Read the model definition and answer for the solid it produces. Units are mm, in the model's axes. Face numbers are marked on the shaded views. A direction names the side the tool comes from. Round coordinates to 2 decimals unless told otherwise and drop trailing zeros. Order: outer loops, then holes, each group sorted by start corner. A loop starts at its lowest first (then second) coordinate and runs counter-clockwise, first axis right, second up. Notation, with made-up numbers: (59, 61.5) -> (93, 61.5) arc R13 ccw to (93, 80.5) -> close; hole circle Ø9 at (74.5, -0.75). An arc over 180 degrees is marked (long way). Use a Markdown table: item, result. Add a question column.
1. For the marked faces 5, 6, 7, 8 and 9, determine the directions among +Z, -Z, +X, -X, +Y, -Y from which every point of the face is accessible in a straight line to the end or side of a thin tool.
2. Given pin 1 (1.2 mm diameter, centred on x = 6, z = 2.5, fed in from +Y); pin 2 (0.9 mm diameter, centred on x = 3.5, z = 3, fed in from +Y); pin 3 (1.2 mm diameter, centred on x = 14, z = 2.5, fed in from +Y), each flat-ended and moving along its own axis, determine where each tip first touches the part or whether it passes through.
3. Section B-B, the plane z = 3 is taken. Give the vertices of the cut face in (x, y).
4. The mould has two halves that part along X. Classify the marked faces 1, 2, 3 and 4: +X half, -X half, draft (parallel to the pull), parting line (faces both ways), or undercut.
5. Section D-D, the plane y = 15.25 is taken. Give the vertices of the cut face in (x, z).
6. Section A-A, the plane y = 10.75 is taken. Give the vertices of the cut face in (x, z).
7. Consider L1, parallel to X at y = 9.25, z = 0.95; L2, parallel to Y at x = 6.25, z = 1.6; L3, parallel to Y at x = 9, z = 3.2. Determine where each line is inside the solid, lowest interval first. Write a range as [from, to].
8. Section C-C, the plane x = 4 is taken. Give the vertices of the cut face in (y, z).
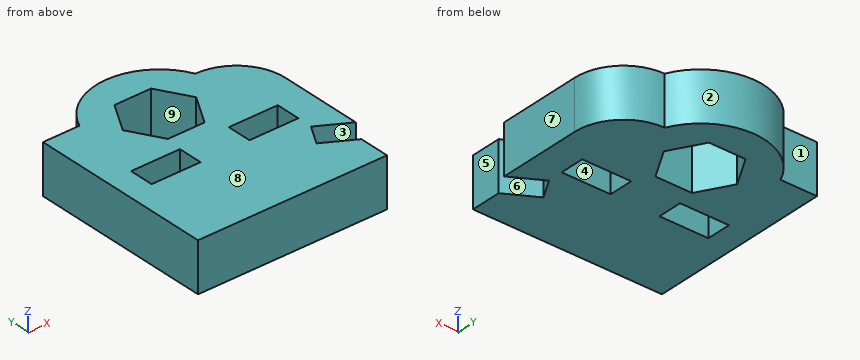
```python
from build123d import *

# Parameters (mm, degrees)
SKETCH1_W           = 4
SKETCH1_H           = 2
BOSS_EXTRUDE1_DEPTH = 4


with BuildPart() as part:
    # Sketch1 → Boss-Extrude1 (new body)
    with BuildSketch(Plane.XY):
        with BuildLine():
            Line((14.475572066, 6), (15.475572066, 7.732050808))
            Line((15.475572066, 7.732050808), (17.939673681, 6.309401077))
            Line((17.939673681, 6.309401077), (17.939673681, 13.142551265))
            ThreePointArc((17.939673681, 13.142551265), (16.768100806, 15.97097839), (13.939673681, 17.142551265))
            ThreePointArc((13.939673681, 17.142551265), (9.2, 20.197069168), (4.460326319, 17.142551265))
            Line((4.460326319, 17.142551265), (1.48, 17.142551265))
            Line((1.48, 17.142551265), (1.48, 2.09107808))
            Line((1.48, 2.09107808), (16.939673681, 2.09107808))
            Line((16.939673681, 2.09107808), (16.939673681, 4.577350269))
            Line((16.939673681, 4.577350269), (14.475572066, 6))
        make_face()
        with Locations((5.5, 9.99107808)):
            Rectangle(SKETCH1_W, SKETCH1_H, mode=Mode.SUBTRACT)
        with Locations((13.5, 9.99107808)):
            Rectangle(SKETCH1_W, SKETCH1_H, mode=Mode.SUBTRACT)
        Polygon((6.2, 14.99107808), (7.7, 12.393001869), (10.7, 12.393001869), (12.2, 14.99107808), (10.7, 17.589154291), (7.7, 17.589154291), align=None, mode=Mode.SUBTRACT)
    extrude(amount=BOSS_EXTRUDE1_DEPTH)


solid = part.part
```
Verdict:
| question | item | result |
|---|---|---|
| 1 | face 5 | +Z, -Z, +X, -Y |
| 1 | face 6 | +Z, -Z, +X |
| 1 | face 7 | +Z, -Z, +X, +Y, -Y |
| 1 | face 8 | +Z, +X, -X, +Y, -Y |
| 1 | face 9 | +Z, -Z |
| 2 | pin 1 | stops at y = 19.5 |
| 2 | pin 2 | stops at y = 17.14 |
| 2 | pin 3 | stops at y = 18.07 |
| 3 | outline | (1.48, 2.09) -> (16.94, 2.09) -> (16.94, 4.58) -> (14.48, 6) -> (15.48, 7.73) -> (17.94, 6.31) -> (17.94, 13.14) arc R4 ccw to (13.94, 17.14) arc R5.2 ccw to (4.46, 17.14) -> (1.48, 17.14) -> close; hole (3.5, 8.99) -> (7.5, 8.99) -> (7.5, 10.99) -> (3.5, 10.99) -> close; hole (6.2, 14.99) -> (7.7, 12.39) -> (10.7, 12.39) -> (12.2, 14.99) -> (10.7, 17.59) -> (7.7, 17.59) -> close; hole (11.5, 8.99) -> (15.5, 8.99) -> (15.5, 10.99) -> (11.5, 10.99) -> close |
| 4 | face 1 | draft |
| 4 | face 2 | parting line |
| 4 | face 3 | undercut |
| 4 | face 4 | undercut |
| 5 | outline | (1.48, 0) -> (6.35, 0) -> (6.35, 4) -> (1.48, 4) -> close; (12.05, 0) -> (17.34, 0) -> (17.34, 4) -> (12.05, 4) -> close |
| 6 | outline | (1.48, 0) -> (3.5, 0) -> (3.5, 4) -> (1.48, 4) -> close; (7.5, 0) -> (11.5, 0) -> (11.5, 4) -> (7.5, 4) -> close; (15.5, 0) -> (17.94, 0) -> (17.94, 4) -> (15.5, 4) -> close |
| 7 | L1 | x = [1.48, 3.5], [7.5, 11.5], [15.5, 17.94] |
| 7 | L2 | y = [2.09, 8.99], [10.99, 14.9], [15.08, 19.28] |
| 7 | L3 | y = [2.09, 12.39], [17.59, 20.19] |
| 8 | outline | (2.09, 0) -> (8.99, 0) -> (8.99, 4) -> (2.09, 4) -> close; (10.99, 0) -> (17.14, 0) -> (17.14, 4) -> (10.99, 4) -> close |
